from build123d import *

# Parameters (mm, degrees)
CROQUIS1_R              = 2.5
SALIENTE_EXTRUIR1_DEPTH = 60
SALIENTE_EXTRUIR2_START = -1
CROQUIS2_R              = 3.75
CROQUIS2_R_2            = 2.5
SALIENTE_EXTRUIR2_DEPTH = 1
CROQUIS5_W              = 3
CROQUIS5_H              = 5.669520972
CORTAR_EXTRUIR1_DEPTH   = 10
CROQUIS6_R              = 0.75
CORTAR_EXTRUIR2_DEPTH   = 4.5
CROQUIS7_W              = 3
CROQUIS7_H              = 6.567565146
CORTAR_EXTRUIR3_DEPTH   = 5
CROQUIS8_R              = 0.75
CORTAR_EXTRUIR4_DEPTH   = 5
CORTAR_EXTRUIR5_DEPTH   = 5


with BuildPart() as part:
    # Croquis1 → Saliente-Extruir1 (new body)
    with BuildSketch(Plane.XY):
        Circle(CROQUIS1_R)
    extrude(amount=SALIENTE_EXTRUIR1_DEPTH)

    # Croquis2 → Saliente-Extruir2 (add)
    with BuildSketch(Plane.XY.offset(18).offset(SALIENTE_EXTRUIR2_START)):
        Circle(CROQUIS2_R)
        Circle(CROQUIS2_R_2, mode=Mode.SUBTRACT)
    extrude(amount=SALIENTE_EXTRUIR2_DEPTH)

    # Croquis5 → Cortar-Extruir1 (cut, symmetric)
    with BuildSketch(Plane.XY.offset(60)):
        Rectangle(CROQUIS5_W, CROQUIS5_H)
    extrude(amount=CORTAR_EXTRUIR1_DEPTH, both=True, mode=Mode.SUBTRACT)

    # Croquis6 → Cortar-Extruir2 (cut, symmetric)
    with BuildSketch(Plane.ZY.offset(-1.5)):
        with Locations((58.5, 0)):
            Circle(CROQUIS6_R)
    extrude(amount=CORTAR_EXTRUIR2_DEPTH, both=True, mode=Mode.SUBTRACT)

    # Croquis7 → Cortar-Extruir3 (cut)
    with BuildSketch(Plane(origin=(0, 0, 0), x_dir=(-1, 0, 0), z_dir=(0, 0, -1))):
        Rectangle(CROQUIS7_W, CROQUIS7_H)
    extrude(amount=-CORTAR_EXTRUIR3_DEPTH, mode=Mode.SUBTRACT)

    # Croquis8 → Cortar-Extruir4 (cut, symmetric)
    with BuildSketch(Plane.ZY.offset(-1.5)):
        with Locations((2, 0)):
            Circle(CROQUIS8_R)
    extrude(amount=CORTAR_EXTRUIR4_DEPTH, both=True, mode=Mode.SUBTRACT)

    # Croquis9 → Cortar-Extruir5 (cut, symmetric)
    with BuildSketch(Plane.ZY.offset(-1.5)):
        with BuildLine():
            Line((0, 2), (2.75, 2))
            ThreePointArc((2.75, 2), (0.75, 0), (2.75, -2))
            Line((2.75, -2), (0, -2))
            Line((0, -2), (0, 2))
        make_face()
    extrude(amount=CORTAR_EXTRUIR5_DEPTH, both=True, mode=Mode.SUBTRACT)


solid = part.part
Geometry check sheet. Reference: the model listing, model coordinates, mm. A direction names the side the tool comes from. Coordinates: 2 decimals unless noted, no trailing zeros. Loops run counter-clockwise (first coordinate to the right, second up) from the corner with the lowest first, then second, coordinate; pieces in that order, holes last. Notation, with made-up numbers: (-20, 63) - (-11, 63) arc R19 ccw to (-11, 89) - close; hole circle Ø3 at (-22.75, 34.5). An arc over 180 degrees is marked (long way). Use one line per item in the form item = value. Start each with the question number.
Item 1: Mould release check, pull along X, two halves, no side actions. Record for faces 6 (the face through (0, 3, 18)), 7 (the face through (-1.5, 0, 3)), 8 (the face through (1.15, -2.22, 10.56)): +X half, -X half, draft (parallel to the pull), parting line (faces both ways), or undercut.
Item 2: Section check A-A, the plane x = 0. Enter the section's corners in (y, z), and give its area (4 significant figures).
Item 3: Thickness scan on probe 1 along Z at (x, y) = (1.8, 0); probe 2 along Y at (x, z) = (-2, 58.5); probe 3 along X at (y, z) = (0, 13.5). Record the ranges inside material, lowest first.
Item 4: Section check C-C, the plane z = 58.5. Enter the section's corners in (x, y), and give its area (3 significant figures).
Item 5: Tool access check on faces 1 (the face through (-1.5, 0, 55)), 2 (the face through (0, 3, 17)), 3 (the face through (0, 0, 5)), 4 (the face through (1.99, 0.03, 1.25)), 5 (the face through (-2.5, 0.1, 38.7)). Record the directions out of +Z, -Z, +X, -X, +Y, -Y that give a thin tool (end or side, any length) a straight path to the whole face; none if there is none.
Item 6: Gauge pin test, flat ends, axial feed: pin 1 (2 mm diameter, centred on y = 0.5, z = 57.5, fed in from -X); pin 2 (2.5 mm diameter, centred on y = 0, z = 2, fed in from +X); pin 3 (2 mm diameter, centred on x = 1.5, y = 2.5, fed in from +Z); pin 4 (2 mm diameter, centred on x = 0.5, y = 2.5, fed in from +Z). Record the tip position at first contact, or that the pin passes through.
Item 7: Section check D-D, the plane y = -3. Enter the section's corners in (x, z), and give its area (3 significant figures).
Item 8: Section check B-B, the plane y = 0. Give the number of separate pieces and of enclosed holes in the cut face, and give its area (3 significant figures).
Computed:
q1.face_6 = draft
q1.face_7 = undercut
q1.face_8 = parting line
q2.outline = (-3.75, 17) - (-2.5, 17) - (-2.5, 5) - (2.5, 5) - (2.5, 17) - (3.75, 17) - (3.75, 18) - (2.5, 18) - (2.5, 50) - (-2.5, 50) - (-2.5, 18) - (-3.75, 18) - close
q2.area = 227.5 mm2
q3.probe_1 = 0.75 to 1.25, 2.75 to 57.75, 59.25 to 60
q3.probe_2 = -1.5 to -0.75, 0.75 to 1.5
q3.probe_3 = -2.5 to 2.5
q4.outline = (-2.38, -0.75) arc R2.5 ccw to (-1.5, -2) - (-1.5, -0.75) - close; (-2.38, 0.75) - (-1.5, 0.75) - (-1.5, 2) arc R2.5 ccw to start; (1.5, -2) arc R2.5 ccw to (2.38, -0.75) - (1.5, -0.75) - close; (1.5, 0.75) - (2.38, 0.75) arc R2.5 ccw to (1.5, 2) - close
q4.area = 2.71 mm2
q5.face_1 = +Z, +Y, -Y
q5.face_2 = -Z
q5.face_3 = -Z, +Y, -Y
q5.face_4 = +X, -X
q5.face_5 = +Z
q6.pin_1 = -2.5
q6.pin_2 = 2.5
q6.pin_3 = 60
q6.pin_4 = 50
q7.outline = (-2.25, 17) - (2.25, 17) - (2.25, 18) - (-2.25, 18) - close
q7.area = 4.50 mm2
q8.separate_pieces = 5
q8.enclosed_holes = 0
q8.area = 250 mm2
